Geometry check sheet. Reference: the model listing, model coordinates, mm. A direction names the side the tool comes from. Give positions to 0.01 mm unless a question says otherwise; leave off trailing zeros. Loops run counter-clockwise (first coordinate to the right, second up) from the corner with the lowest first, then second, coordinate; pieces in that order, holes last. Notation, with made-up numbers: (16.5, 34) -> (20.5, 34) arc R24 ccw to (20.5, 68) -> close; hole circle Ø7 at (11, 61). An arc over 180 degrees is marked (long way). One line per question, with ' | ' between items.
from build123d import *

# Parameters (mm, degrees)
F0_W     = 50.8
F0_H     = 50.8
F1_DEPTH = 50.8
F2_R     = 14.126259
F3_DEPTH = 50.8
F4_W     = 25.4
F4_H     = 25.4
F5_DEPTH = 12.7
F6_R     = 12.7
F7_DEPTH = 12.7


with BuildPart() as f1:
    # F0 (on Front) → F1 (new body)
    with BuildSketch(Plane.XZ):
        with Locations((-25.4, 25.4)):
            Rectangle(F0_W, F0_H)
    extrude(amount=F1_DEPTH)

    # F2 (on face) → F3 (cut)
    with BuildSketch(Plane.XZ.offset(50.8)):
        with Locations((-25.4, 25.4)):
            Circle(F2_R)
    extrude(amount=-F3_DEPTH, mode=Mode.SUBTRACT)

    # F4 (on face) → F5 (join)
    with BuildSketch(Plane(origin=(0, 0, 0), x_dir=(1, 0, 0), z_dir=(0, 0, -1))):
        with Locations((-25.4, 25.4)):
            Rectangle(F4_W, F4_H)
    extrude(amount=F5_DEPTH)

    # F6 (on face) → F7 (join)
    with BuildSketch(Plane(origin=(-50.8, 0, 0), x_dir=(0, -1, 0), z_dir=(-1, 0, 0))):
        with Locations((25.4, 25.4)):
            Circle(F6_R)
    extrude(amount=F7_DEPTH)


solid = f1.part
Item 1: Sectioned sample at D-D (x = -7). Record the cut outline in (y, z), plus the area to 3 significant figures.
Result:
outline: (-50.8, 0) -> (0, 0) -> (0, 50.8) -> (-50.8, 50.8) -> close | area: 2,580 mm2
Item 2: Sectioned sample at C-C (x = -25.4). Record the cut outline in (y, z).
Result:
outline: (-50.8, 0) -> (-38.1, 0) -> (-38.1, -12.7) -> (-12.7, -12.7) -> (-12.7, 0) -> (0, 0) -> (0, 11.27) -> (-50.8, 11.27) -> close; (-50.8, 39.53) -> (0, 39.53) -> (0, 50.8) -> (-50.8, 50.8) -> close
Item 3: Sectioned sample at B-B (y = -25.4). Record the cut outline in (x, z).
Result:
outline: (-63.5, 12.7) -> (-50.8, 12.7) -> (-50.8, 0) -> (-38.1, 0) -> (-38.1, -12.7) -> (-12.7, -12.7) -> (-12.7, 0) -> (0, 0) -> (0, 50.8) -> (-50.8, 50.8) -> (-50.8, 38.1) -> (-63.5, 38.1) -> close; hole circle Ø28.25 at (-25.4, 25.4)
Item 4: Sectioned sample at A-A (z = 25.4). Record the cut outline in (x, y), plus the area to 3 significant figures.
Result:
outline: (-63.5, -38.1) -> (-50.8, -38.1) -> (-50.8, -50.8) -> (-39.53, -50.8) -> (-39.53, 0) -> (-50.8, 0) -> (-50.8, -12.7) -> (-63.5, -12.7) -> close; (-11.27, -50.8) -> (0, -50.8) -> (0, 0) -> (-11.27, 0) -> close | area: 1,470 mm2
Item 5: Scan lines: probe 1 along Z at (x, y) = (-25, -30); probe 2 along X at (y, z) = (-18, 25); probe 3 along Z at (x, y) = (-25, -10). Record each from-to range of solid material in increasing order.
Result:
probe 1: -12.7 to 11.28, 39.52 to 50.8 | probe 2: -63.5 to -39.52, -11.28 to 0 | probe 3: 0 to 11.28, 39.52 to 50.8
Item 6: Depth check by flat-ended pin: pin 1 Ø6.5 at (y, z) = (-23.5, -8) entering from +X; pin 2 Ø10 at (y, z) = (-25.5, -6) entering from -X; pin 3 Ø1.5 at (x, y) = (-46, -19.5) entering from -Z. Enter the tip coordinate at first touch or a pass-through.
Result:
pin 1: x = -12.7 | pin 2: x = -38.1 | pin 3: z = 0
Item 7: Release check for a two-part mould opening along X. For faces 6 (the face through (-18.88, -25.76, 12.87)), 7 (the face through (-26, -26, -12.7)), 8 (the face through (0, -25, 25)) record: pulls with the +X half, pulls with the -X half, needs draft (parallel to the pull), parting line crosses it, or undercut.
Result:
face 6: undercut | face 7: needs draft | face 8: pulls with the +X half
Item 8: Set-up check for faces 1 (the face through (-26, -12.7, -6)), 2 (the face through (-26, -38.1, -6)), 3 (the face through (-38.1, -25, -6)), 4 (the face through (-50.8, -19, 14)), 5 (the face through (-12.7, -25, -6)): record each of +Z, -Z, +X, -X, +Y, -Y from which the full face is reachable in a straight line by a thin tool's end or side.
Result:
face 1: -Z, +X, -X, +Y | face 2: -Z, +X, -X, -Y | face 3: -Z, -X, +Y, -Y | face 4: -X | face 5: -Z, +X, +Y, -Y
